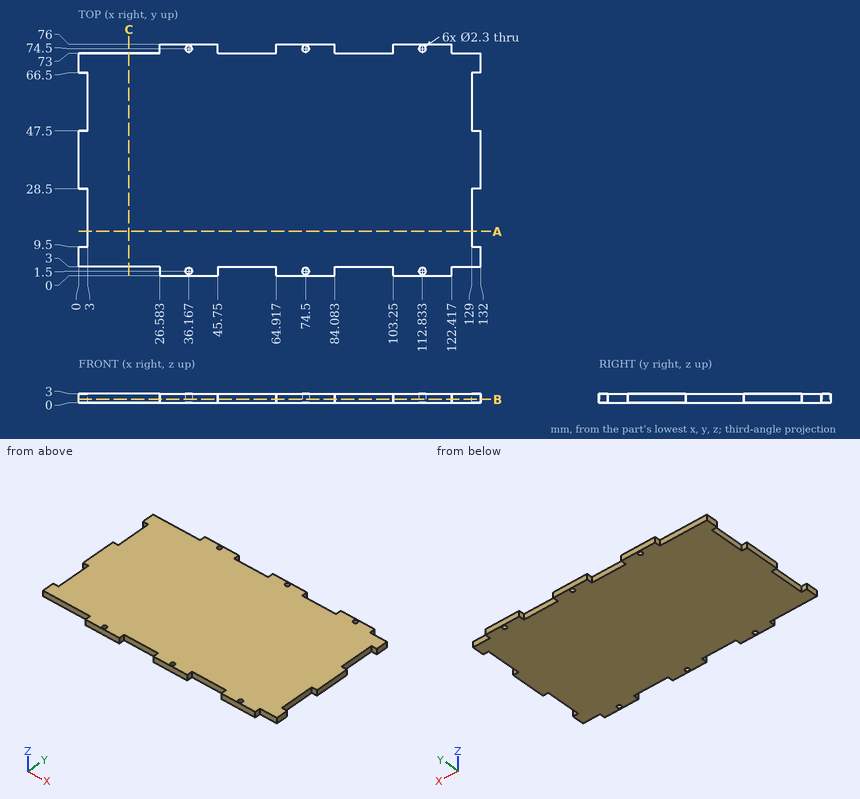
Design review of the part shown in the three views and the two pictorial views. Dimensions are in mm from the part's minimum x, y and z. Give positions to 0.01 mm unless a question says otherwise; leave off trailing zeros. Loops run counter-clockwise (first coordinate to the right, second up) from the corner with the lowest first, then second, coordinate; pieces in that order, holes last. Notation, with made-up numbers: M 61.5,8.5 L 73.5,8.5 A12 ccw 73.5,19.5 Z; hole C 57.5,53 d6. An arc over 180 degrees is marked long. Answer as a JSON object with one key per item and string values.
Item 1: Wall thickness on line 1 along X through (y, z) = (74.5, 0.8); line 2 along Y through (x, z) = (74.5, 0.95); line 3 along X through (y, z) = (15, 2.65): over which ranges is each line inside the solid? List them lowest first.
Output values:
{"line 1": "x = 26.58 to 35.02, 37.32 to 45.75, 64.92 to 73.35, 75.65 to 84.08, 103.25 to 111.68, 113.98 to 122.42", "line 2": "y = 0 to 0.35, 2.65 to 73.35, 75.65 to 76", "line 3": "x = 3 to 129"}
Item 2: We need section C-C (x = 16.5). State the section outline as (y, z) points.
Output values:
{"outline": "M 3,0 L 73,0 L 73,3 L 3,3 Z"}
Item 3: We need section A-A (y = 14.5). State the section outline as (x, z) points.
Output values:
{"outline": "M 3,0 L 129,0 L 129,3 L 3,3 Z"}
Item 4: For P1, Ø0.9, axis at x = 2, z = 2, coming from the +Y side; P2, Ø1, axis at x = 58.5, z = 1.5, coming from the -Y side; P3, Ø2.5, axis at x = 36.17, y = 1.5, coming from the +Z side; P4, Ø0.9, axis at y = 19, z = 2, coming from the -X side, all flat-tipped, find the tip position at first contact; note any pin that passes through.
Output values:
{"P1": "stops at y = 73", "P2": "stops at y = 3", "P3": "stops at z = 3", "P4": "stops at x = 3"}
Item 5: We need section B-B (z = 1.1). Count the separate pieces of the cut face and the enclosed holes in it, and give its area (3 significant figures).
Output values:
{"separate pieces": "1", "enclosed holes": "6", "area": "9,330 mm2"}
